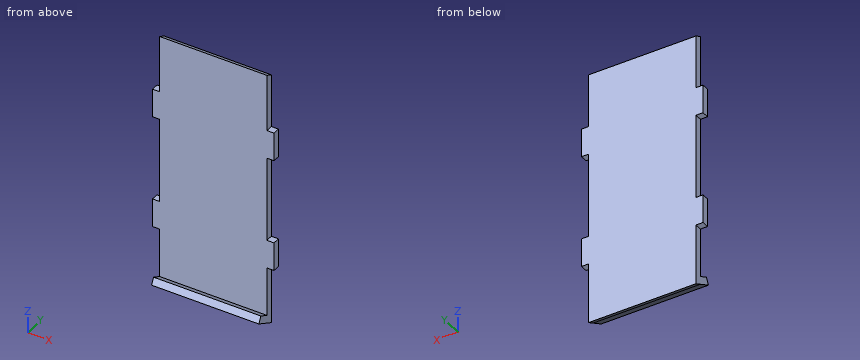
from build123d import *

# Parameters (mm, degrees)
F1_DEPTH = 3.175
F3_DEPTH = 43.942
F5_DEPTH = 76.2
F6_DEPTH = 48.1697538


# Not quite as in the source:
# - a feature names something its author has since deleted; it is built from what else it names


with BuildPart() as f1:
    # F0 (on Front) → F1 (new body)
    with BuildSketch(Plane.XZ):
        Polygon((-34.9639124011, -57.0107064), (9.4471751978, -57.0107064), (13.2058413989, -57.0107064), (13.2058413989, -31.6107064), (16.3808413989, -31.6107064), (16.3808413989, -18.9107064), (13.2058413989, -18.9107064), (13.2058413989, 18.9107064), (16.3808413989, 18.9107064), (16.3808413989, 31.6107064), (13.2058413989, 31.6107064), (13.2058413989, 57.0107064), (-34.9639124011, 57.0107064), (-34.9639124011, 31.6107064), (-38.1389124011, 31.6107064), (-38.1389124011, 18.9107064), (-34.9639124011, 18.9107064), (-34.9639124011, -18.9107064), (-38.1389124011, -18.9107064), (-38.1389124011, -31.6107064), (-34.9639124011, -31.6107064), align=None)
    extrude(amount=F1_DEPTH)

    # F2 (on face) → F3 (join)
    with BuildSketch(Plane(origin=(-34.9639124011, 0, 0), x_dir=(0, -1, 0), z_dir=(-1, 0, 0))):
        Polygon((0, -58.6279720227), (3.175, -57.0107064), (8.8332357394, -54.1285425744), (7.3921538265, -51.2994247047), (0, -55.0648030547), align=None)
    extrude(amount=-F3_DEPTH)

    # F4 (on face) → F5 (cut)
    with BuildSketch(Plane(origin=(-34.9639124011, 0, 0), x_dir=(0, -1, 0), z_dir=(-1, 0, 0))):
        Polygon((0, 55.3934407773), (3.175, 57.0107064), (0, 57.0107064), align=None)
    extrude(amount=-F5_DEPTH, mode=Mode.SUBTRACT)

    # F2 (on face) → F6 (join)
    with BuildSketch(Plane(origin=(-34.9639124011, 0, 0), x_dir=(0, -1, 0), z_dir=(-1, 0, 0))):
        Polygon((0, -58.6279720227), (3.175, -57.0107064), (8.8332357394, -54.1285425744), (7.3921538265, -51.2994247047), (0, -55.0648030547), align=None)
    extrude(amount=-F6_DEPTH)


solid = f1.part
Design review of the part built by this model. Coordinates are the model's own, in mm. Give positions to 0.01 mm unless a question says otherwise; leave off trailing zeros. Write each loop counter-clockwise with the first axis right and the second up, starting at its lowest first coordinate (ties: lowest second). Pieces come first, ordered by that corner, then holes. Notation, with made-up numbers: M 30,2 L 83,2 A24 ccw 83,22 Z; hole C 64.25,19.25 d6. An arc over 180 degrees is marked long. Answer as a JSON object with one key per item and string values. Group by question number.
1) Clearance check with flat-ended pins moving along their axes: pin 1 Ø2.5 at (x, y) = (-36, -1.5) entering from -Z; pin 2 Ø5 at (x, y) = (-11.5, -4) entering from +Z; pin 3 Ø1.6 at (y, z) = (-2, 1) entering from -X; pin 4 Ø1 at (x, y) = (-37, -1.5) entering from +Z. State where each tip first meets the part, or that it passes through.
2) We need section A-A (x = 4). Give the boundary of the cut face in (y, z) (3 decimals), and give its area (3 significant figures).
3) We need section B-B (z = 47). Give the boundary of the cut face in (x, y) (3 decimals).
4) For line 1 along Y through (x, z) = (-9, 26.5) (3 decimals); line 2 along X through (y, z) = (-3, -3); line 3 along Y through (x, z) = (-33, -52) (3 decimals), list the stretches that pass through material, from the lowest coordinate up.
5) We need section C-C (y = -2). Give the boundary of the cut face in (x, z), and give its area (3 significant figures).
6) We need section D-D (z = 28). Give the boundary of the cut face in (x, y) (3 decimals), and give its area (3 significant figures).
Answer key:
{
 "1": {"pin 1": "stops at z = -58.22", "pin 2": "stops at z = 57.01", "pin 3": "stops at x = -34.96", "pin 4": "stops at z = 31.61"},
 "2": {"outline": "M -8.833,-54.129 L 0,-58.628 L 0,55.393 L -3.175,57.011 L -3.175,-53.448 L -7.392,-51.299 Z", "area": "380 mm²"},
 "3": {"outline": "M -34.964,-3.175 L 13.206,-3.175 L 13.206,0 L -34.964,0 Z"},
 "4": {"line 1": "y = -3.175 to 0", "line 2": "x = -34.96 to 13.21", "line 3": "y = -7.749 to -6.017, -3.175 to 0"},
 "5": {"outline": "M -38.14,-31.61 L -34.96,-31.61 L -34.96,-57.61 L 13.21,-57.61 L 13.21,-31.61 L 16.38,-31.61 L 16.38,-18.91 L 13.21,-18.91 L 13.21,18.91 L 16.38,18.91 L 16.38,31.61 L 13.21,31.61 L 13.21,56.41 L -34.96,56.41 L -34.96,31.61 L -38.14,31.61 L -38.14,18.91 L -34.96,18.91 L -34.96,-18.91 L -38.14,-18.91 Z", "area": "5,650 mm²"},
 "6": {"outline": "M -38.139,-3.175 L 16.381,-3.175 L 16.381,0 L -38.139,0 Z", "area": "173 mm²"}
}
